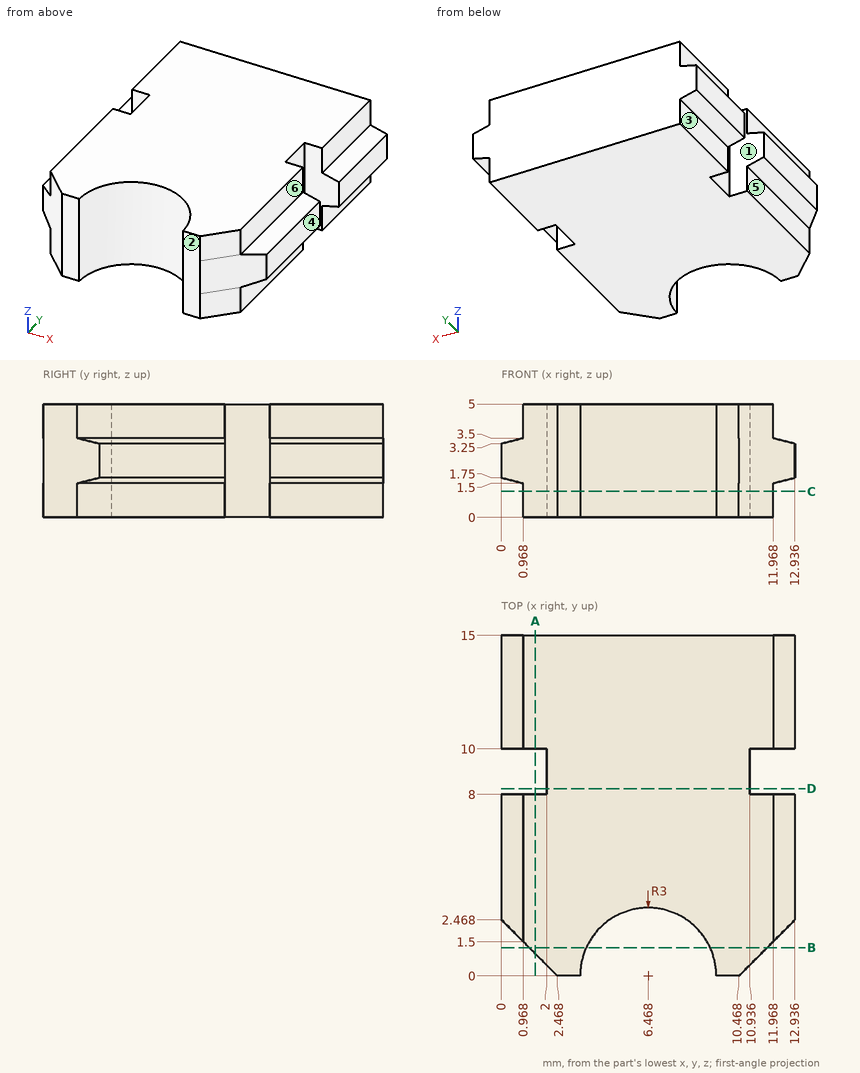
Geometry check sheet. Reference: drawing and pictorial views, mm from the part's lowest x, y, z. A direction names the side the tool comes from. Round coordinates to 2 decimals unless told otherwise and drop trailing zeros. Write each loop counter-clockwise with the first axis right and the second up, starting at its lowest first coordinate (ties: lowest second). Pieces come first, ordered by that corner, then holes.
(1) Section check C-C (z = 1.15). Enter the section's corners in (x, y).
Returned:
outline: (0.97, 1.5) - (2.47, 0) - (3.47, 0) arc R3 cw to (9.47, 0) - (10.47, 0) - (11.97, 1.5) - (11.97, 8) - (10.94, 8) - (10.94, 10) - (11.97, 10) - (11.97, 15) - (0.97, 15) - (0.97, 10) - (2, 10) - (2, 8) - (0.97, 8) - close
(2) Mould release check, pull along Y, two halves, no side actions. Record for the marked faces 1, 2 and 3: pulls with the +Y half, pulls with the -Y half, needs draft (parallel to the pull), parting line crosses it, or undercut.
Returned:
face 1: undercut
face 2: pulls with the -Y half
face 3: needs draft
(3) Section check D-D (y = 8.25). Enter the section's corners in (x, z), plus the area to 3 significant figures.
Returned:
outline: (2, 0) - (10.94, 0) - (10.94, 5) - (2, 5) - close
area: 44.7 mm2
(4) Section check B-B (y = 1.25). Enter the section's corners in (x, z) (1 decimal).
Returned:
outline: (1.2, 0) - (3.7, 0) - (3.7, 5) - (1.2, 5) - close; (9.2, 0) - (11.7, 0) - (11.7, 5) - (9.2, 5) - close
(5) Section check A-A (x = 1.5). Enter the section's corners in (y, z).
Returned:
outline: (0.97, 0) - (8, 0) - (8, 5) - (0.97, 5) - close; (10, 0) - (15, 0) - (15, 5) - (10, 5) - close
(6) Depth check by flat-ended pin: pin 1 Ø0.8 at (y, z) = (4.5, 4.5) entering from -X; pin 2 Ø1 at (y, z) = (9, 3.5) entering from +X; pin 3 Ø1.6 at (x, z) = (12, 3) entering from -Y. Enter the tip coordinate at first touch or a pass-through.
Returned:
pin 1: stops at x = 0.97
pin 2: stops at x = 10.94
pin 3: stops at y = 0.73
(7) Access from +Z, -Z, +X, -X, +Y, -Y to the whole of each face (thin tool, end or side, straight path). Record for the marked faces 4, 5 and 6.
Returned:
face 4: +Z, -Z, +X, +Y, -Y
face 5: -Z, -X, +Y, -Y
face 6: +Z, +X, +Y, -Y
(8) Material ranges on line 1 (X direction, y = 9, z = 1.9); line 2 (X direction, y = 5.5, z = 4.55); line 3 (X direction, y = 2.5, z = 4.65) (1 decimal), recorded low to high.
Returned:
line 1: x = 2 to 10.94
line 2: x = 0.97 to 11.97
line 3: x = 1 to 4.8, 8.1 to 12
